Part model, mm, in its own coordinate system. A direction names the side the tool comes from. Round coordinates to 2 decimals unless told otherwise and drop trailing zeros. Order: outer loops, then holes, each group sorted by start corner. A loop starts at its lowest first (then second) coordinate and runs counter-clockwise, first axis right, second up. Notation, with made-up numbers: (-1, 38.5) -> (28, 38.5) arc R25 ccw to (28, 72.5) -> close; hole circle Ø2 at (35, -39). An arc over 180 degrees is marked (long way). Use CSV: the item, a comma, the result in double quotes.
```python
from build123d import *

# Parameters (mm, degrees)
SKETCH1_W               = 64.75
SKETCH1_H               = 84.325
SKETCH1_R               = 1.35
BOSS_EXTRUDE1_DEPTH     = 25.4
CUT_EXTRUDE1_DEPTH      = 82.335102547
SKETCH5_W               = 58.925
SKETCH5_H               = 20.6375
CUT_EXTRUDE3_DEPTH      = 82.335102547
BOSS_EXTRUDE2_START     = 4.7625
SKETCH1_3_W             = 6.75
SKETCH1_3_H             = 6.75
SKETCH1_3_R             = 1.35
SKETCH1_3_H_2           = 3.175
BOSS_EXTRUDE2_DEPTH     = 9.525
CUT_EXTRUDE6_DEPTH      = 55.65443286
CUT_EXTRUDE6_DEPTH_BACK = 55.65443286
SKETCH7_W               = 26.65
SKETCH7_H               = 62.1
SKETCH8_W               = 40.894
SKETCH8_H               = 33.274
SKETCH8_W_2             = 8
SKETCH8_H_2             = 8
BOSS_EXTRUDE3_DEPTH     = 11.5
SKETCH8_3_W             = 8
SKETCH8_3_H             = 8
CUT_EXTRUDE7_DEPTH      = 9.5
CUT_EXTRUDE8_DEPTH      = 6
SKETCH9_W               = 26.65
SKETCH9_H               = 86.865
CUT_EXTRUDE9_DEPTH      = 6
CUT_EXTRUDE10_DEPTH     = 84.258730216
SKETCH11_W              = 64.75
SKETCH11_H              = 84.325
CUT_EXTRUDE11_DEPTH     = 86.930007316
BOSS_EXTRUDE4_DEPTH     = 40.894
SKETCH15_W              = 7.376
SKETCH15_H              = 9.883286215
SKETCH15_W_2            = 20
SKETCH15_H_2            = 9.293713785
CUT_EXTRUDE12_DEPTH     = 79.999970514
CUT_EXTRUDE14_START     = -33.274
CUT_EXTRUDE14_DEPTH     = 80.122835409
FILLET1_R               = 3.175
FILLET2_R               = 2.54
SKETCH22_W              = 9.202496002
SKETCH22_H              = 15.787790907
CUT_EXTRUDE17_DEPTH     = 87.575023929


with BuildPart() as part:
    # Sketch1 → Boss-Extrude1 (new body)
    with BuildSketch(Plane(origin=(0, 0, 0), x_dir=(1, 0, 0), z_dir=(0, 1, 0))):
        Rectangle(SKETCH1_W, SKETCH1_H)
        with Locations(Location((-29, 10.2125, 0), (0, 0, 270))):
            Circle(SKETCH1_R, mode=Mode.SUBTRACT)
        with Locations(Location((29, 10.2125, 0), (0, 0, 270))):
            Circle(SKETCH1_R, mode=Mode.SUBTRACT)
        with Locations(Location((-29, -38.7875, 0), (0, 0, 270))):
            Circle(SKETCH1_R, mode=Mode.SUBTRACT)
        with Locations(Location((29, -38.7875, 0), (0, 0, 270))):
            Circle(SKETCH1_R, mode=Mode.SUBTRACT)
    extrude(amount=BOSS_EXTRUDE1_DEPTH)

    # Sketch3 → Cut-Extrude1 (cut, through all)
    with BuildSketch(Plane(origin=(32.375, 0, 0), x_dir=(0, 0, -1), z_dir=(1, 0, 0))):
        Polygon((42.1625, 18.034), (23.1125, 18.669), (23.1125, 12.7), (42.1625, 12.7), align=None)
    extrude(amount=-CUT_EXTRUDE1_DEPTH, mode=Mode.SUBTRACT)

    # Sketch5 → Cut-Extrude3 (cut, through all)
    with BuildSketch(Plane(origin=(32.375, 0, 0), x_dir=(0, 0, -1), z_dir=(1, 0, 0))):
        with Locations((-12.7, 15.08125)):
            Rectangle(SKETCH5_W, SKETCH5_H)
    extrude(amount=-CUT_EXTRUDE3_DEPTH, mode=Mode.SUBTRACT)

    # Sketch1<3> → Boss-Extrude2 (add)
    # profile 1 of 6: a face of its own
    with BuildSketch(Plane(origin=(0, 0, 0), x_dir=(1, 0, 0), z_dir=(0, 1, 0)).offset(BOSS_EXTRUDE2_START)):
        with Locations((29, -38.7875)):
            Rectangle(SKETCH1_3_W, SKETCH1_3_H)
        with Locations(Location((29, -38.7875, 0), (0, 0, 90))):
            Circle(SKETCH1_3_R, mode=Mode.SUBTRACT)
    # profile 2 of 6: a face of its own
    with BuildSketch(Plane(origin=(0, 0, 0), x_dir=(1, 0, 0), z_dir=(0, 1, 0)).offset(BOSS_EXTRUDE2_START)):
        with Locations((-29, -38.7875)):
            Rectangle(SKETCH1_3_W, SKETCH1_3_H)
        with Locations(Location((-29, -38.7875, 0), (0, 0, 90))):
            Circle(SKETCH1_3_R, mode=Mode.SUBTRACT)
    # profile 3 of 6: a face of its own
    with BuildSketch(Plane(origin=(0, 0, 0), x_dir=(1, 0, 0), z_dir=(0, 1, 0)).offset(BOSS_EXTRUDE2_START)):
        with Locations((-29, 10.2125)):
            Rectangle(SKETCH1_3_W, SKETCH1_3_H)
        with Locations(Location((-29, 10.2125, 0), (0, 0, 90))):
            Circle(SKETCH1_3_R, mode=Mode.SUBTRACT)
    # profile 4 of 6: a face of its own
    with BuildSketch(Plane(origin=(0, 0, 0), x_dir=(1, 0, 0), z_dir=(0, 1, 0)).offset(BOSS_EXTRUDE2_START)):
        with Locations((29, 10.2125)):
            Rectangle(SKETCH1_3_W, SKETCH1_3_H)
        with Locations(Location((29, 10.2125, 0), (0, 0, 90))):
            Circle(SKETCH1_3_R, mode=Mode.SUBTRACT)
    # profile 5 of 6: a face of its own
    with BuildSketch(Plane(origin=(0, 0, 0), x_dir=(1, 0, 0), z_dir=(0, 1, 0)).offset(BOSS_EXTRUDE2_START)):
        with Locations((-29, 15.175)):
            Rectangle(SKETCH1_3_W, SKETCH1_3_H_2)
    # profile 6 of 6: a face of its own
    with BuildSketch(Plane(origin=(0, 0, 0), x_dir=(1, 0, 0), z_dir=(0, 1, 0)).offset(BOSS_EXTRUDE2_START)):
        with Locations((29, 15.175)):
            Rectangle(SKETCH1_3_W, SKETCH1_3_H_2)
    extrude(amount=BOSS_EXTRUDE2_DEPTH)

    # Sketch7 → Cut-Extrude6 (cut, two sides: drawn at the far end of the back side and taken through both)
    with BuildSketch(Plane(origin=(0, 12.7, 0), x_dir=(1, 0, 0), z_dir=(0, 1, 0)).offset(-CUT_EXTRUDE6_DEPTH_BACK)):
        with Locations((0, -1.5875)):
            Rectangle(SKETCH7_W, SKETCH7_H)
    extrude(amount=CUT_EXTRUDE6_DEPTH + CUT_EXTRUDE6_DEPTH_BACK, mode=Mode.SUBTRACT)

    # Sketch8 → Boss-Extrude3 (add)
    with BuildSketch(Plane.XZ):
        with Locations((0, 58.7995)):
            Rectangle(SKETCH8_W, SKETCH8_H)
        with Locations((-10.541, 50.7985)):
            Rectangle(SKETCH8_W_2, SKETCH8_H_2, mode=Mode.SUBTRACT)
        with Locations((10.541, 50.7985)):
            Rectangle(SKETCH8_W_2, SKETCH8_H_2, mode=Mode.SUBTRACT)
        with Locations((-10.541, 66.1655)):
            Rectangle(SKETCH8_W_2, SKETCH8_H_2, mode=Mode.SUBTRACT)
        with Locations((10.541, 66.1655)):
            Rectangle(SKETCH8_W_2, SKETCH8_H_2, mode=Mode.SUBTRACT)
    extrude(amount=-BOSS_EXTRUDE3_DEPTH)

    # Sketch8<3> → Cut-Extrude7 (cut)
    # profile 1 of 4: a face of its own
    with BuildSketch(Plane.XZ):
        Polygon((-16.637, 47.4965), (-16.637, 44.7025), (-4.445, 44.7025), (-4.445, 46.7984953), (-2.8575, 46.7984953), (-2.8575, 54.7985047), (-4.445, 54.7985047), (-4.445, 56.8945), (-16.637, 56.8945), (-16.637, 54.1005), (-17.399, 54.1005), (-17.399, 47.4965), align=None)
        with Locations((-10.541, 50.7985)):
            Rectangle(SKETCH8_3_W, SKETCH8_3_H, mode=Mode.SUBTRACT)
    # profile 2 of 4: a face of its own
    with BuildSketch(Plane.XZ):
        Polygon((4.445, 56.8945), (4.445, 54.7985047), (2.8575, 54.7985047), (2.8575, 46.7984953), (4.445, 46.7984953), (4.445, 44.7025), (16.637, 44.7025), (16.637, 47.4965), (17.399, 47.4965), (17.399, 54.1005), (16.637, 54.1005), (16.637, 56.8945), align=None)
        with Locations((10.541, 50.7985)):
            Rectangle(SKETCH8_3_W, SKETCH8_3_H, mode=Mode.SUBTRACT)
    # profile 3 of 4: a face of its own
    with BuildSketch(Plane.XZ):
        Polygon((-16.637, 72.2615), (-16.637, 69.4675), (-17.399, 69.4675), (-17.399, 62.8635), (-16.637, 62.8635), (-16.637, 60.0695), (-4.445, 60.0695), (-4.445, 62.1654953), (-2.8575, 62.1654953), (-2.8575, 70.1655047), (-4.445, 70.1655047), (-4.445, 72.2615), align=None)
        with Locations((-10.541, 66.1655)):
            Rectangle(SKETCH8_3_W, SKETCH8_3_H, mode=Mode.SUBTRACT)
    # profile 4 of 4: a face of its own
    with BuildSketch(Plane.XZ):
        Polygon((4.445, 72.2615), (4.445, 70.1655047), (2.8575, 70.1655047), (2.8575, 62.1654953), (4.445, 62.1654953), (4.445, 60.0695), (16.637, 60.0695), (16.637, 62.8635), (17.399, 62.8635), (17.399, 69.4675), (16.637, 69.4675), (16.637, 72.2615), align=None)
        with Locations((10.541, 66.1655)):
            Rectangle(SKETCH8_3_W, SKETCH8_3_H, mode=Mode.SUBTRACT)
    extrude(amount=-CUT_EXTRUDE7_DEPTH, mode=Mode.SUBTRACT)

    # Sketch8<4> → Cut-Extrude8 (cut)
    with BuildSketch(Plane.XZ):
        Polygon((-4.445, 46.7984953), (-4.445, 44.7025), (4.445, 44.7025), (4.445, 46.7984953), (2.8575, 46.7984953), (2.8575, 54.7985047), (4.445, 54.7985047), (4.445, 56.8945), (16.637, 56.8945), (16.637, 60.0695), (4.445, 60.0695), (4.445, 62.1654953), (2.8575, 62.1654953), (2.8575, 70.1655047), (4.445, 70.1655047), (4.445, 72.2615), (-4.445, 72.2615), (-4.445, 70.1655047), (-2.8575, 70.1655047), (-2.8575, 62.1654953), (-4.445, 62.1654953), (-4.445, 60.0695), (-16.637, 60.0695), (-16.637, 56.8945), (-4.445, 56.8945), (-4.445, 54.7985047), (-2.8575, 54.7985047), (-2.8575, 46.7984953), align=None)
    extrude(amount=-CUT_EXTRUDE8_DEPTH, mode=Mode.SUBTRACT)

    # Sketch9 → Cut-Extrude9 (cut)
    with BuildSketch(Plane.XZ):
        with Locations((0, 1.27)):
            Rectangle(SKETCH9_W, SKETCH9_H)
    extrude(amount=-CUT_EXTRUDE9_DEPTH, mode=Mode.SUBTRACT)

    # Sketch10 → Cut-Extrude10 (cut, through all)
    with BuildSketch(Plane(origin=(0, 11.5, 0), x_dir=(1, 0, 0), z_dir=(0, 1, 0))):
        Polygon((-0.762, -56.8945), (0.762, -56.8945), (0.762, -51.0525), (2.032, -51.0525), (0, -45.9725), (-2.032, -51.0525), (-0.762, -51.0525), align=None)
        Polygon((-0.762, -65.9115), (-0.762, -60.0695), (0.762, -60.0695), (0.762, -65.9115), (2.032, -65.9115), (0, -70.9915), (-2.032, -65.9115), align=None)
    extrude(amount=-CUT_EXTRUDE10_DEPTH, mode=Mode.SUBTRACT)

    # Sketch11 → Cut-Extrude11 (cut, through all)
    with BuildSketch(Plane.XZ):
        Rectangle(SKETCH11_W, SKETCH11_H)
    extrude(amount=-CUT_EXTRUDE11_DEPTH, mode=Mode.SUBTRACT)

    # Sketch14 → Boss-Extrude4 (add)
    with BuildSketch(Plane(origin=(20.447, 0, 0), x_dir=(0, 0, -1), z_dir=(1, 0, 0))):
        with BuildLine():
            Line((-38.942699076, 7.350099538), (-39.3685, 2.3))
            Line((-39.3685, 2.3), (-36.819487459, 2.3))
            Line((-36.819487459, 2.3), (-36.043786215, 11.5))
            Line((-36.043786215, 11.5), (-42.1625, 11.5))
            Line((-42.1625, 11.5), (-42.1625, 7.350099538))
            ThreePointArc((-42.1625, 7.350099538), (-40.552599538, 8.96), (-38.942699076, 7.350099538))
        make_face()
    extrude(amount=-BOSS_EXTRUDE4_DEPTH)

    # Sketch15 → Cut-Extrude12 (cut, through all)
    with BuildSketch(Plane(origin=(0, 11.5, 0), x_dir=(1, 0, 0), z_dir=(0, 1, 0))):
        with Locations((16.759, -31.102143108)):
            Rectangle(SKETCH15_W, SKETCH15_H)
        with Locations((-16.759, -31.102143108)):
            Rectangle(SKETCH15_W, SKETCH15_H)
        with Locations((0, -40.690643108)):
            Rectangle(SKETCH15_W_2, SKETCH15_H_2)
        with Locations((0, -40.690643108)):
            Rectangle(SKETCH15_W_2, SKETCH15_H_2)
    extrude(amount=-CUT_EXTRUDE12_DEPTH, mode=Mode.SUBTRACT)

    # Sketch18 → Cut-Extrude14 (cut, through all)
    with BuildSketch(Plane.XY.offset(75.4365).offset(CUT_EXTRUDE14_START)):
        Polygon((18.542, 1.569), (18.542, 3.319), (-18.542, 3.319), (-18.542, 1.569), (-16.637, 1.569), (-16.637, 0), (16.637, 0), (16.637, 1.569), align=None)
    extrude(amount=CUT_EXTRUDE14_DEPTH, mode=Mode.SUBTRACT)

    # Fillet1
    fillet1_edges = [part.edges().sort_by_distance(p)[0] for p in [
        (-15.2235, 11.5, 36.043786215),
        (15.2235, 11.5, 36.043786215),
    ]]
    fillet(fillet1_edges, radius=FILLET1_R)

    # Fillet2
    # the kernel refuses this fillet: 2.54 mm, written as the material it takes off along each edge
    with BuildSketch(Plane(origin=(-3.11459751, 2.3, 39.3685), x_dir=(0, 0, -1), z_dir=(-1, 0, 0)), Plane(origin=(27.33240249, 2.3, 39.3685), x_dir=(0, 0, -1), z_dir=(-1, 0, 0))) as fillet2_piece_1:
        with BuildLine():
            CenterArc((2.762416328, -2.531019325), FILLET2_R, 94.819514659, 90)
            Line((0.231397003, -2.744423112), (0.180776616, -2.748691188))
            Line((0.180776616, -2.748691188), (-0.050620387, -0.004268076))
            Line((-0.050620387, -0.004268076), (0, 0.0508))
            ThreePointArc((0, 0.0508), (1.27450627, 0.0508), (2.544744465, 0.050620387))
            Line((2.544744465, 0.050620387), (2.549012541, 0))
        make_face()
    extrude(amount=24.217804979, mode=Mode.SUBTRACT)

    # Sketch22 → Cut-Extrude17 (cut, through all)
    with BuildSketch(Plane.ZY.offset(20.447)):
        with Locations((37.561251999, 7.893895454)):
            Rectangle(SKETCH22_W, SKETCH22_H)
    extrude(amount=-CUT_EXTRUDE17_DEPTH, mode=Mode.SUBTRACT)


solid = part.part
```
(1) Cut at C-C, the plane z = 59.5. Give the cut face in (x, y).
Reply:
outline,"(-20.45, 0) -> (-16.64, 0) -> (-16.64, 1.57) -> (-18.54, 1.57) -> (-18.54, 3.32) -> (-16.64, 3.32) -> (-16.64, 6) -> (16.64, 6) -> (16.64, 3.32) -> (18.54, 3.32) -> (18.54, 1.57) -> (16.64, 1.57) -> (16.64, 0) -> (20.45, 0) -> (20.45, 11.5) -> (-20.45, 11.5) -> close"
(2) Probe probe 1 along Z at (x, y) = (12.5, 10); probe 2 along Z at (x, y) = (15, 7.25); probe 3 along X at (y, z) = (4.75, 50). List the from-to ranges inside material, lowest first. Write a range as [from, to].
Reply:
probe 1,"[42.16, 46.8], [54.8, 62.17], [70.17, 75.44]"
probe 2,"[42.16, 44.7], [56.89, 60.07], [72.26, 75.44]"
probe 3,"[-20.45, -17.4], [17.4, 20.45]"
(3) Pull direction X, two halves, no side cores. Call faces 6 (the face through (16.637, 6, 46)), 7 (the face through (0, 7, 75.436)): released by +X, released by -X, zero draft, split by the parting line, or undercut.
Reply:
face 6,"undercut"
face 7,"zero draft"
(4) Drop flat-ended pins along their axis: P1, Ø5, axis at x = 9, z = 48.5, coming from the -Y side; P2, Ø0.5, axis at x = 4, y = 7.5, coming from the -Z side. Give the stop position or say it passes through.
Reply:
P1,"y = 9.5"
P2,"z = 45.34"
(5) Cut at B-B, the plane y = 2.75. Give the cut face in (x, z), then the cut area to 3 significant figures.
Reply:
outline,"(-20.45, 42.16) -> (-18.54, 42.16) -> (-18.54, 75.44) -> (-20.45, 75.44) -> close; (18.54, 42.16) -> (20.45, 42.16) -> (20.45, 75.44) -> (18.54, 75.44) -> close"
area,"127 mm2"
(6) Cut at A-A, the plane x = -8.5. Give the cut face in (y, z).
Reply:
outline,"(3.32, 72.26) -> (9.5, 72.26) -> (9.5, 70.17) -> (11.5, 70.17) -> (11.5, 75.44) -> (3.32, 75.44) -> close; (6, 56.89) -> (9.5, 56.89) -> (9.5, 54.8) -> (11.5, 54.8) -> (11.5, 62.17) -> (9.5, 62.17) -> (9.5, 60.07) -> (6, 60.07) -> close; (9.5, 45.34) -> (11.5, 45.34) -> (11.5, 46.8) -> (9.5, 46.8) -> close"
(7) Which spindle directions (+Z, -Z, +X, -X, +Y, -Y) get a long thin tool onto all of the face, cutting with end or side? Do faces 1 (the face through (16.637, 1, 72)), 2 (the face through (-0.762, 9, 63)), 3 (the face through (-4.445, 8, 56)), 4 (the face through (-10, 9, 43)), 5 (the face through (10, 8, 60.07)). Say none if no direction does.
Reply:
face 1,"+Z, -Z, -Y"
face 2,"+Y, -Y"
face 3,"-Z, -Y"
face 4,"-Z, +Y, -Y"
face 5,"-Y"
(8) Cut at D-D, the plane z = 65. State how many separate pieces and enclosed holes the cut face has, then the cut area to 3 significant figures.
Reply:
separate pieces,"4"
enclosed holes,"0"
area,"115 mm2"
